Source: CAD feature listing. Evaluate the final solid. Frame: model axes, mm. Face numbers are marked on the shaded views. Give positions to 0.01 mm unless a question says otherwise; leave off trailing zeros. Loops run counter-clockwise (first coordinate to the right, second up) from the corner with the lowest first, then second, coordinate; pieces in that order, holes last. Notation, with made-up numbers: (31.5, 10) - (65.5, 10) arc R20 cw to (65.5, 39) - close; hole circle Ø9 at (-25, 44). An arc over 180 degrees is marked (long way). Write each question's results on one line, items separated by ' | '. Start each with the question number.
(1) Material intervals for line 1 along X through (y, z) = (29, -17.5); line 2 along X through (y, z) = (1.6, -110); line 3 along Y through (x, z) = (6, -87), sorted ascending. Write a range as [from, to].
(2) Cut plane B-B on x = 48. Give the number of separate pieces and of enclosed holes in the cut face, then the cut area to 3 significant figures.
(3) Contact query for flat-ended pins moving along their axis: pin 1 (4 mm diameter, centred on x = 45.5, z = -37.5, fed in from +Y); pin 2 (0.6 mm diameter, centred on y = 1, z = -105.5, fed in from +X). Output: stop coordinate, or through.
(4) Cut plane A-A on y = 25. Return the cut outline in (x, z), then the cut area to 3 significant figures.
(5) Pull-direction query (X, two-part tool) for the marked faces 1, 2 and 3; classes: pulls with the +X half, pulls with the -X half, needs draft (parallel to the pull), parting line crosses it, or undercut.
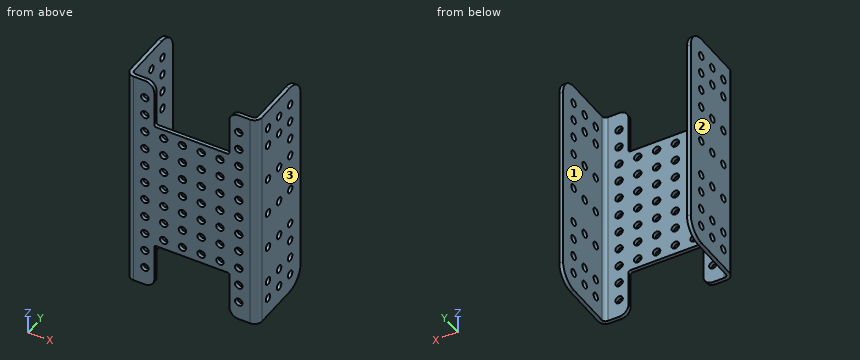
from build123d import *

# Parameters (mm, degrees)
SKETCH1_W                      = 66
SKETCH1_H                      = 120
BOSS_EXTRUDE1_DEPTH            = 2
SKETCH2_R                      = 2
CUT_EXTRUDE1_DEPTH             = 137.967149346
EDGE_FLANGE1_STRIP_W           = 12
EDGE_FLANGE1_STRIP_H           = 2
EDGE_FLANGE1_STRIP_CUT_DEPTH   = 120
EDGE_FLANGE1_STRIP_2_W         = 12
EDGE_FLANGE1_STRIP_2_H         = 2
EDGE_FLANGE1_STRIP_CUT_2_DEPTH = 120
EDGE_FLANGE1_DEPTH             = 120
EDGE_FLANGE1_BEND_DEPTH        = 120
SKETCH24_W                     = 40
SKETCH24_H                     = 25
CUT_EXTRUDE6_DEPTH             = 143.804061567
FILLET1_R                      = 10
FILLET2_R                      = 5
FILLET3_R                      = 1
SKETCH25_R                     = 2
CUT_EXTRUDE8_DEPTH             = 145.294837052


# Sheet-metal steps are written as plain solids
with BuildPart() as part:
    # Sketch1 → Boss-Extrude1 (new body)
    with BuildSketch(Plane(origin=(0, 0, 0), x_dir=(1, 0, 0), z_dir=(0, 1, 0))):
        with Locations((33, 60)):
            Rectangle(SKETCH1_W, SKETCH1_H)
    extrude(amount=BOSS_EXTRUDE1_DEPTH)

    # Sketch2 → Cut-Extrude1 (cut, through all)
    with BuildSketch(Plane(origin=(0, 2, 0), x_dir=(1, 0, 0), z_dir=(0, 1, 0))):
        with Locations(Location((8, 110, 0), (0, 0, 270))):
            Circle(SKETCH2_R)
        with Locations(Location((18, 110, 0), (0, 0, 270))):
            Circle(SKETCH2_R)
        with Locations(Location((28, 110, 0), (0, 0, 270))):
            Circle(SKETCH2_R)
        with Locations(Location((38, 110, 0), (0, 0, 270))):
            Circle(SKETCH2_R)
        with Locations(Location((48, 110, 0), (0, 0, 270))):
            Circle(SKETCH2_R)
        with Locations(Location((58, 110, 0), (0, 0, 270))):
            Circle(SKETCH2_R)
        with Locations(Location((18, 100, 0), (0, 0, 270))):
            Circle(SKETCH2_R)
        with Locations(Location((28, 100, 0), (0, 0, 270))):
            Circle(SKETCH2_R)
        with Locations(Location((38, 100, 0), (0, 0, 270))):
            Circle(SKETCH2_R)
        with Locations(Location((48, 100, 0), (0, 0, 270))):
            Circle(SKETCH2_R)
        with Locations(Location((58, 100, 0), (0, 0, 270))):
            Circle(SKETCH2_R)
        with Locations(Location((18, 90, 0), (0, 0, 270))):
            Circle(SKETCH2_R)
        with Locations(Location((28, 90, 0), (0, 0, 270))):
            Circle(SKETCH2_R)
        with Locations(Location((38, 90, 0), (0, 0, 270))):
            Circle(SKETCH2_R)
        with Locations(Location((48, 90, 0), (0, 0, 270))):
            Circle(SKETCH2_R)
        with Locations(Location((58, 90, 0), (0, 0, 270))):
            Circle(SKETCH2_R)
        with Locations(Location((18, 80, 0), (0, 0, 270))):
            Circle(SKETCH2_R)
        with Locations(Location((28, 80, 0), (0, 0, 270))):
            Circle(SKETCH2_R)
        with Locations(Location((38, 80, 0), (0, 0, 270))):
            Circle(SKETCH2_R)
        with Locations(Location((48, 80, 0), (0, 0, 270))):
            Circle(SKETCH2_R)
        with Locations(Location((58, 80, 0), (0, 0, 270))):
            Circle(SKETCH2_R)
        with Locations(Location((18, 70, 0), (0, 0, 270))):
            Circle(SKETCH2_R)
        with Locations(Location((28, 70, 0), (0, 0, 270))):
            Circle(SKETCH2_R)
        with Locations(Location((38, 70, 0), (0, 0, 270))):
            Circle(SKETCH2_R)
        with Locations(Location((48, 70, 0), (0, 0, 270))):
            Circle(SKETCH2_R)
        with Locations(Location((58, 70, 0), (0, 0, 270))):
            Circle(SKETCH2_R)
        with Locations(Location((18, 60, 0), (0, 0, 270))):
            Circle(SKETCH2_R)
        with Locations(Location((28, 60, 0), (0, 0, 270))):
            Circle(SKETCH2_R)
        with Locations(Location((38, 60, 0), (0, 0, 270))):
            Circle(SKETCH2_R)
        with Locations(Location((48, 60, 0), (0, 0, 270))):
            Circle(SKETCH2_R)
        with Locations(Location((58, 60, 0), (0, 0, 270))):
            Circle(SKETCH2_R)
        with Locations(Location((18, 50, 0), (0, 0, 270))):
            Circle(SKETCH2_R)
        with Locations(Location((28, 50, 0), (0, 0, 270))):
            Circle(SKETCH2_R)
        with Locations(Location((38, 50, 0), (0, 0, 270))):
            Circle(SKETCH2_R)
        with Locations(Location((48, 50, 0), (0, 0, 270))):
            Circle(SKETCH2_R)
        with Locations(Location((58, 50, 0), (0, 0, 270))):
            Circle(SKETCH2_R)
        with Locations(Location((18, 40, 0), (0, 0, 270))):
            Circle(SKETCH2_R)
        with Locations(Location((28, 40, 0), (0, 0, 270))):
            Circle(SKETCH2_R)
        with Locations(Location((38, 40, 0), (0, 0, 270))):
            Circle(SKETCH2_R)
        with Locations(Location((48, 40, 0), (0, 0, 270))):
            Circle(SKETCH2_R)
        with Locations(Location((58, 40, 0), (0, 0, 270))):
            Circle(SKETCH2_R)
        with Locations(Location((18, 30, 0), (0, 0, 270))):
            Circle(SKETCH2_R)
        with Locations(Location((28, 30, 0), (0, 0, 270))):
            Circle(SKETCH2_R)
        with Locations(Location((38, 30, 0), (0, 0, 270))):
            Circle(SKETCH2_R)
        with Locations(Location((48, 30, 0), (0, 0, 270))):
            Circle(SKETCH2_R)
        with Locations(Location((58, 30, 0), (0, 0, 270))):
            Circle(SKETCH2_R)
        with Locations(Location((18, 20, 0), (0, 0, 270))):
            Circle(SKETCH2_R)
        with Locations(Location((28, 20, 0), (0, 0, 270))):
            Circle(SKETCH2_R)
        with Locations(Location((38, 20, 0), (0, 0, 270))):
            Circle(SKETCH2_R)
        with Locations(Location((48, 20, 0), (0, 0, 270))):
            Circle(SKETCH2_R)
        with Locations(Location((58, 20, 0), (0, 0, 270))):
            Circle(SKETCH2_R)
        with Locations(Location((18, 10, 0), (0, 0, 270))):
            Circle(SKETCH2_R)
        with Locations(Location((28, 10, 0), (0, 0, 270))):
            Circle(SKETCH2_R)
        with Locations(Location((38, 10, 0), (0, 0, 270))):
            Circle(SKETCH2_R)
        with Locations(Location((48, 10, 0), (0, 0, 270))):
            Circle(SKETCH2_R)
        with Locations(Location((58, 10, 0), (0, 0, 270))):
            Circle(SKETCH2_R)
        with Locations(Location((8, 100, 0), (0, 0, 270))):
            Circle(SKETCH2_R)
        with Locations(Location((8, 90, 0), (0, 0, 270))):
            Circle(SKETCH2_R)
        with Locations(Location((8, 80, 0), (0, 0, 270))):
            Circle(SKETCH2_R)
        with Locations(Location((8, 70, 0), (0, 0, 270))):
            Circle(SKETCH2_R)
        with Locations(Location((8, 60, 0), (0, 0, 270))):
            Circle(SKETCH2_R)
        with Locations(Location((8, 50, 0), (0, 0, 270))):
            Circle(SKETCH2_R)
        with Locations(Location((8, 40, 0), (0, 0, 270))):
            Circle(SKETCH2_R)
        with Locations(Location((8, 30, 0), (0, 0, 270))):
            Circle(SKETCH2_R)
        with Locations(Location((8, 20, 0), (0, 0, 270))):
            Circle(SKETCH2_R)
        with Locations(Location((8, 10, 0), (0, 0, 270))):
            Circle(SKETCH2_R)
    extrude(amount=-CUT_EXTRUDE1_DEPTH, mode=Mode.SUBTRACT)

    # Edge-Flange1 strip (across the edge) → Edge-Flange1 strip cut (cut)
    with BuildSketch(Plane(origin=(0, 2, -120), x_dir=(1, 0, 0), z_dir=(0, 0, 1))):
        with Locations((-4, -1)):
            Rectangle(EDGE_FLANGE1_STRIP_W, EDGE_FLANGE1_STRIP_H)
    extrude(amount=EDGE_FLANGE1_STRIP_CUT_DEPTH, mode=Mode.SUBTRACT)

    # Edge-Flange1 strip 2 (across the edge) → Edge-Flange1 strip cut 2 (cut)
    with BuildSketch(Plane(origin=(66, 2, 0), x_dir=(-1, 0, 0), z_dir=(0, 0, -1))):
        with Locations((-4, -1)):
            Rectangle(EDGE_FLANGE1_STRIP_2_W, EDGE_FLANGE1_STRIP_2_H)
    extrude(amount=EDGE_FLANGE1_STRIP_CUT_2_DEPTH, mode=Mode.SUBTRACT)

    # Edge-Flange1 section (across the edge) → Edge-Flange1 (add)
    with BuildSketch(Plane(origin=(0, 2, -120), x_dir=(1, 0, 0), z_dir=(0, 0, 1))):
        with BuildLine():
            Line((-2, 2), (-2, 37))
            Line((-2, 37), (0, 37))
            Line((0, 37), (0, 2))
            ThreePointArc((0, 2), (0.585786438, 0.585786438), (2, 0))
            Line((2, 0), (2, -2))
            ThreePointArc((2, -2), (-0.828427125, -0.828427125), (-2, 2))
        make_face()
    extrude(amount=EDGE_FLANGE1_DEPTH)

    # Edge-Flange1 section 2 (across the edge) → Edge-Flange1 bend (add)
    with BuildSketch(Plane(origin=(66, 2, 0), x_dir=(-1, 0, 0), z_dir=(0, 0, -1))):
        with BuildLine():
            Line((-2, 2), (-2, 37))
            Line((-2, 37), (0, 37))
            Line((0, 37), (0, 2))
            ThreePointArc((0, 2), (0.585786438, 0.585786438), (2, 0))
            Line((2, 0), (2, -2))
            ThreePointArc((2, -2), (-0.828427125, -0.828427125), (-2, 2))
        make_face()
    extrude(amount=EDGE_FLANGE1_BEND_DEPTH)

    # Sketch24 → Cut-Extrude6 (cut, through all)
    with BuildSketch(Plane(origin=(0, 2, 0), x_dir=(1, 0, 0), z_dir=(0, 1, 0))):
        with Locations((33, 107.5)):
            Rectangle(SKETCH24_W, SKETCH24_H)
        with Locations((33, 12.5)):
            Rectangle(SKETCH24_W, SKETCH24_H)
    extrude(amount=-CUT_EXTRUDE6_DEPTH, mode=Mode.SUBTRACT)

    # Fillet1
    fillet1_edges = [part.edges().sort_by_distance(p)[0] for p in [
        (-1, 39, -120),
        (-1, 39, 0),
        (67, 39, 0),
        (67, 39, -120),
    ]]
    fillet(fillet1_edges, radius=FILLET1_R)

    # Fillet2
    fillet2_edges = [part.edges().sort_by_distance(p)[0] for p in [
        (13, 1, -120),
        (53, 1, -120),
        (53, 1, 0),
        (13, 1, 0),
    ]]
    fillet(fillet2_edges, radius=FILLET2_R)

    # Fillet3
    fillet3_edges = [part.edges().sort_by_distance(p)[0] for p in [
        (13, 1, -95),
        (53, 1, -95),
        (13, 1, -25),
        (53, 1, -25),
    ]]
    fillet(fillet3_edges, radius=FILLET3_R)

    # Sketch25 → Cut-Extrude8 (cut, through all)
    with BuildSketch(Plane(origin=(68, 0, 0), x_dir=(0, 0, -1), z_dir=(1, 0, 0))):
        with Locations(Location((10, 29.5, 0), (0, 0, 90))):
            Circle(SKETCH25_R)
        with Locations(Location((20, 29.5, 0), (0, 0, 90))):
            Circle(SKETCH25_R)
        with Locations(Location((30, 29.5, 0), (0, 0, 90))):
            Circle(SKETCH25_R)
        with Locations(Location((40, 29.5, 0), (0, 0, 90))):
            Circle(SKETCH25_R)
        with Locations(Location((60, 29.5, 0), (0, 0, 90))):
            Circle(SKETCH25_R)
        with Locations(Location((80, 29.5, 0), (0, 0, 90))):
            Circle(SKETCH25_R)
        with Locations(Location((90, 29.5, 0), (0, 0, 90))):
            Circle(SKETCH25_R)
        with Locations(Location((100, 29.5, 0), (0, 0, 90))):
            Circle(SKETCH25_R)
        with Locations(Location((110, 29.5, 0), (0, 0, 90))):
            Circle(SKETCH25_R)
        with Locations(Location((20, 19.5, 0), (0, 0, 90))):
            Circle(SKETCH25_R)
        with Locations(Location((40, 19.5, 0), (0, 0, 90))):
            Circle(SKETCH25_R)
        with Locations(Location((60, 19.5, 0), (0, 0, 90))):
            Circle(SKETCH25_R)
        with Locations(Location((80, 19.5, 0), (0, 0, 90))):
            Circle(SKETCH25_R)
        with Locations(Location((100, 19.5, 0), (0, 0, 90))):
            Circle(SKETCH25_R)
        with Locations(Location((110, 19.5, 0), (0, 0, 90))):
            Circle(SKETCH25_R)
        with Locations(Location((20, 9.5, 0), (0, 0, 90))):
            Circle(SKETCH25_R)
        with Locations(Location((40, 9.5, 0), (0, 0, 90))):
            Circle(SKETCH25_R)
        with Locations(Location((60, 9.5, 0), (0, 0, 90))):
            Circle(SKETCH25_R)
        with Locations(Location((80, 9.5, 0), (0, 0, 90))):
            Circle(SKETCH25_R)
        with Locations(Location((100, 9.5, 0), (0, 0, 90))):
            Circle(SKETCH25_R)
        with Locations(Location((110, 9.5, 0), (0, 0, 90))):
            Circle(SKETCH25_R)
        with Locations(Location((10, 19.5, 0), (0, 0, 90))):
            Circle(SKETCH25_R)
        with Locations(Location((10, 9.5, 0), (0, 0, 90))):
            Circle(SKETCH25_R)
    extrude(amount=-CUT_EXTRUDE8_DEPTH, mode=Mode.SUBTRACT)


solid = part.part
Ans:
1) line 1: [-2, 0], [66, 68] | line 2: [-1.2, 6], [10, 13], [53, 56], [60, 67.2] | line 3: [0, 2]
2) separate pieces: 8 | enclosed holes: 0 | area: 84.0 mm^2
3) pin 1: y = 2 | pin 2: x = 66.95
4) outline: (-2, -120) - (0, -120) - (0, 0) - (-2, 0) - close; (66, -120) - (68, -120) - (68, 0) - (66, 0) - close | area: 480 mm^2
5) face 1: undercut | face 2: pulls with the -X half | face 3: pulls with the +X half
